The listing builds one solid part. Answer for the finished solid, in the listing's coordinates (mm). A direction names the side the tool comes from. Coordinates: 2 decimals unless noted, no trailing zeros. Write each loop counter-clockwise with the first axis right and the second up, starting at its lowest first coordinate (ties: lowest second). Pieces come first, ordered by that corner, then holes.
```python
from build123d import *

# Parameters (mm, degrees)
F0_W     = 24
F0_H     = 24
F0_W_2   = 22
F0_H_2   = 22
F1_DEPTH = 25
F2_W     = 3
F2_H     = 3
F3_DEPTH = 1
F4_W     = 3
F4_H     = 3
F5_DEPTH = 1


with BuildPart() as f1:
    # F0 (on Top) → F1 (new body)
    with BuildSketch(Plane.XY):
        Rectangle(F0_W, F0_H)
        Rectangle(F0_W_2, F0_H_2, mode=Mode.SUBTRACT)
    extrude(amount=F1_DEPTH)

    # F2 (on face) → F3 (cut, through all)
    with BuildSketch(Plane.XZ.offset(12)):
        with Locations((-4.5, 19.5)):
            Rectangle(F2_W, F2_H)
        with Locations((4.5, 19.5)):
            Rectangle(F2_W, F2_H)
    extrude(amount=-F3_DEPTH, mode=Mode.SUBTRACT)

    # F4 (on face) → F5 (cut, through all)
    with BuildSketch(Plane(origin=(0, 12, 0), x_dir=(-1, 0, 0), z_dir=(0, 1, 0))):
        with Locations((-6, 6.5)):
            Rectangle(F4_W, F4_H)
        with Locations((-6, 12.5)):
            Rectangle(F4_W, F4_H)
        with Locations((-6, 18.5)):
            Rectangle(F4_W, F4_H)
        with Locations((6, 18.5)):
            Rectangle(F4_W, F4_H)
        with Locations((6, 12.5)):
            Rectangle(F4_W, F4_H)
        with Locations((6, 6.5)):
            Rectangle(F4_W, F4_H)
    extrude(amount=-F5_DEPTH, mode=Mode.SUBTRACT)


solid = f1.part
```
(1) Find the intervals of material crossed by probe 1 along Y at (x, z) = (1.5, 1.5); probe 2 along Y at (x, z) = (6, 6), in increasing order.
(2) Which of the six approach directions +Z, -Z, +X, -X, +Y, -Y give full straight-line access (tool end or side, diameter ignored) to faces 4 (the flat face through (7.5, 11.5, 12.5)), 5 (the flat face through (4.5, -11.5, 21)), 6 (the flat face through (-12, 0, 12)), 7 (the flat face through (0, -12, 12)), 8 (the flat face through (0, -11, 12))?
(3) Section B-B, the plane x = -4 is taken. Write down the section's boundary in (y, z).
(4) For a pull along Z with two mould halves and no side action, classify faces 1 (the flat face through (-0.9, -11.5, 0)), 2 (the flat face through (3, -11.5, 19.5)), 3 (the flat face through (-0.9, -11.5, 25)) as pulls with the +Z half, pulls with the -Z half, needs draft (parallel to the pull), parting line crosses it, or undercut.
(5) Section A-A, the plane y = 10 is taken. Write down the section's boundary in (x, z), plus the area to 3 significant figures.
(6) This flat-tipped pin is pushed along its axis until it touches: pin 1 (1.1 mm diameter, centred on x = -4.5, y = -11.5, fed in from -Z). Where does it stop, or does it pass through?
(7) Section C-C, the plane z = 15 is taken. Write down the section's boundary in (x, y), plus the area to 3 significant figures.
Solution:
1. probe 1: y = -12 to -11, 11 to 12
1. probe 2: y = -12 to -11
2. face 4: +Y
2. face 5: -Y
2. face 6: +Z, -Z, -X, +Y, -Y
2. face 7: +Z, -Z, +X, -X, -Y
2. face 8: +Z, -Z
3. outline: (-12, 0) - (-11, 0) - (-11, 18) - (-12, 18) - close; (-12, 21) - (-11, 21) - (-11, 25) - (-12, 25) - close; (11, 0) - (12, 0) - (12, 25) - (11, 25) - close
4. face 1: pulls with the -Z half
4. face 2: undercut
4. face 3: pulls with the +Z half
5. outline: (-12, 0) - (-11, 0) - (-11, 25) - (-12, 25) - close; (11, 0) - (12, 0) - (12, 25) - (11, 25) - close
5. area: 50.0 mm2
6. pin 1: stops at z = 0
7. outline: (-12, -12) - (12, -12) - (12, 12) - (-12, 12) - close; hole (-11, -11) - (11, -11) - (11, 11) - (-11, 11) - close
7. area: 92.0 mm2
